Part print with two shaded views. Sizes in mm from the minimum x, y, z corner. Give positions to 0.01 mm unless a question says otherwise; leave off trailing zeros. Write each loop counter-clockwise with the first axis right and the second up, starting at its lowest first coordinate (ties: lowest second). Pieces come first, ordered by that corner, then holes. Notation, with made-up numbers: (50, 25) - (59, 25) arc R29 cw to (59, 55) - close; hole circle Ø7 at (14.25, 21). An arc over 180 degrees is marked (long way). Answer as a JSON object with one key per item and string values.
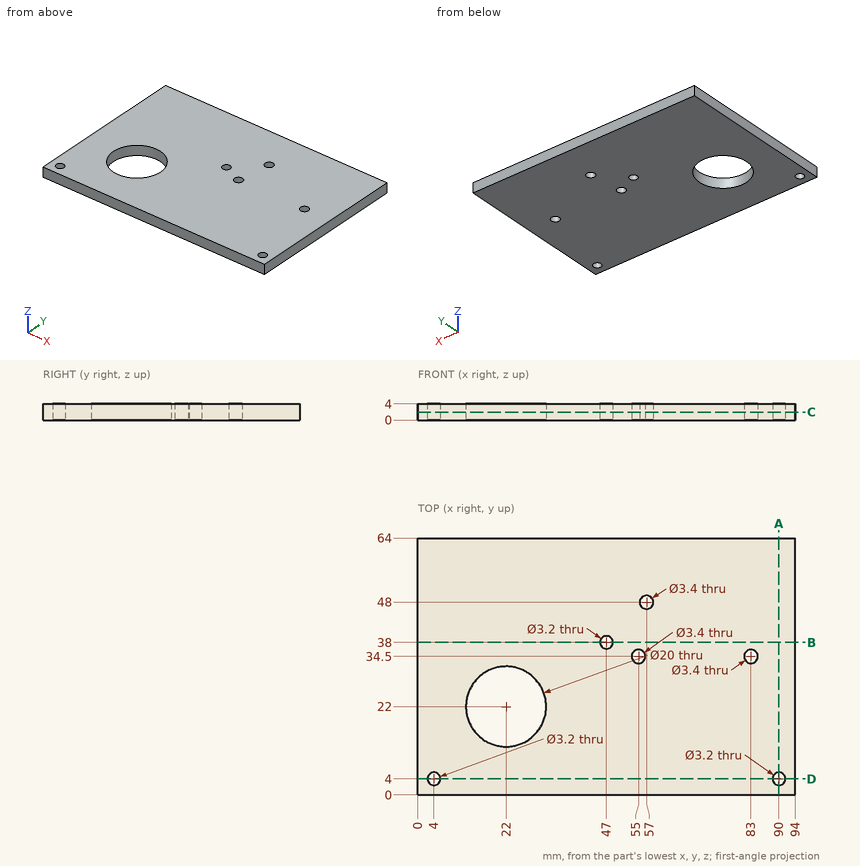
(1) Saw through at C-C, the plane z = 2. Give the cut face in (x, y).
Answer key:
{"outline": "(0, 0) - (94, 0) - (94, 64) - (0, 64) - close; hole circle Ø3.2 at (4, 4); hole circle Ø20 at (22, 22); hole circle Ø3.2 at (47, 38); hole circle Ø3.4 at (55, 34.5); hole circle Ø3.4 at (57, 48); hole circle Ø3.4 at (83, 34.5); hole circle Ø3.2 at (90, 4)"}
(2) Saw through at A-A, the plane x = 90. Give the cut face in (y, z), and give its area (3 significant figures).
Answer key:
{"outline": "(0, 0) - (2.4, 0) - (2.4, 4) - (0, 4) - close; (5.6, 0) - (64, 0) - (64, 4) - (5.6, 4) - close", "area": "243 mm²"}
(3) Saw through at D-D, the plane y = 4. Give the cut face in (x, z), and give its area (3 significant figures).
Answer key:
{"outline": "(0, 0) - (2.4, 0) - (2.4, 4) - (0, 4) - close; (5.6, 0) - (88.4, 0) - (88.4, 4) - (5.6, 4) - close; (91.6, 0) - (94, 0) - (94, 4) - (91.6, 4) - close", "area": "350 mm²"}
(4) Flat gauge pins, fed straight in: P1, Ø3.5, axis at x = 4, y = 4, coming from the +Z side; P2, Ø1.9, axis at x = 90, y = 4, coming from the +Z side. Where does each tip first touch, or does it go through?
Answer key:
{"P1": "stops at z = 4", "P2": "passes through"}
(5) Saw through at B-B, the plane y = 38. Give the cut face in (x, z).
Answer key:
{"outline": "(0, 0) - (45.4, 0) - (45.4, 4) - (0, 4) - close; (48.6, 0) - (94, 0) - (94, 4) - (48.6, 4) - close"}
(6) Probe L1, parallel to X at y = 34.5, z = 2.9; L2, parallel to X at y = 4, z = 1.6; L3, parallel to X at y = 48, z = 2.1. List the from-to ranges inside material, lowest first. Write a range as [from, to].
Answer key:
{"L1": "x = [0, 53.3], [56.7, 81.3], [84.7, 94]", "L2": "x = [0, 2.4], [5.6, 88.4], [91.6, 94]", "L3": "x = [0, 55.3], [58.7, 94]"}
